from build123d import *

# Parameters (mm, degrees)
F0_R     = 5.5
F1_DEPTH = 9
F3_DEPTH = 9
F4_R     = 7
F5_DEPTH = 9


with BuildPart() as f1:
    # F0 (on Top) → F1 (new body)
    with BuildSketch(Plane.XY):
        with BuildLine():
            Line((-46, 15), (-46, 0))
            ThreePointArc((-46, 0), (-42.192388, -9.192388), (-33, -13))
            Line((-33, -13), (0, -13))
            ThreePointArc((0, -13), (9.192388, -9.192388), (13, 0))
            Line((13, 0), (13, 15))
            Line((13, 15), (-46, 15))
        make_face()
        with Locations((-33, 0)):
            Circle(F0_R, mode=Mode.SUBTRACT)
        Circle(F0_R, mode=Mode.SUBTRACT)
    extrude(amount=F1_DEPTH)

    # F2 (on face) → F3 (join)
    with BuildSketch(Plane(origin=(0, 15, 0), x_dir=(-1, 0, 0), z_dir=(0, 1, 0))):
        Polygon((46, 0), (46, 9), (-20.313708, 75.313708), (-42.941125, 52.686292), (-13, 0), align=None)
    extrude(amount=F3_DEPTH)

    # F4 (on face) → F5 (join)
    with BuildSketch(Plane(origin=(47.813708, 0, 47.813708), x_dir=(0.707107, 0, -0.707107), z_dir=(0.707107, 0, 0.707107))):
        with BuildLine():
            Line((-6.890873, 15), (-6.890873, 24))
            Line((-6.890873, 24), (-38.890873, 24))
            Line((-38.890873, 24), (-38.890873, 15))
            Line((-38.890873, 15), (-38.890875, -5))
            ThreePointArc((-38.890875, -5), (-22.890875, -21), (-6.890875, -5))
            Line((-6.890875, -5), (-6.890873, 15))
        make_face()
        with Locations((-22.890875, -5)):
            Circle(F4_R, mode=Mode.SUBTRACT)
    extrude(amount=F5_DEPTH)


solid = f1.part
For this review, take the finished solid that the model builds, in its own axes (mm). A direction names the side the tool comes from. Round coordinates to 2 decimals unless told otherwise and drop trailing zeros. Order: outer loops, then holes, each group sorted by start corner. A loop starts at its lowest first (then second) coordinate and runs counter-clockwise, first axis right, second up. Notation, with made-up numbers: (37, 49.5) -> (72, 49.5) arc R21 cw to (72, 71.5) -> close; hole circle Ø6 at (30, -4.75). An arc over 180 degrees is marked (long way). Put each result on its own line as item: value.
Q1. Machinability: for faces 4 (the flat face through (-17, 1, 9)), 5 (the flat face through (-16, 5, 0)), 6 (the flat face through (28.955, 1.252, 66.673)), 7 (the flat face through (13, 7, 4)), 8 (the cylindrical face through (30.84, -9.26, 71.07)), which of the approach directions +Z, -Z, +X, -X, +Y, -Y give a long, thin tool a straight path to every point of the face, cutting with its end or side? Answer none if there is none.
Check result:
face 4: +Z, +X, -X, -Y
face 5: -Z, +X, -X, +Y, -Y
face 6: -Z, -X, -Y
face 7: +Z, -Z, +X, -Y
face 8: none
Q2. For probe 1 along Y at (x, z) = (-33, 7); probe 2 along Z at (x, y) = (-16, -1); probe 3 along Z at (x, y) = (43, -12.5), list the stretches that pass through material, from the lowest coordinate up. Write a range as [from, to].
Check result:
probe 1: [-13, -5.5], [5.5, 24]
probe 2: [0, 9]
probe 3: [55.39, 65.36]
Q3. Add section D-D on z = 33.5. Write out the cut boundary in (x, y).
Check result:
outline: (-21.5, 15) -> (32.04, 15) -> (32.04, 24) -> (-21.5, 24) -> close
Q4. Add section A-A on y = 10. Write out the cut boundary in (x, z), plus the area to 3 significant figures.
Check result:
outline: (-46, 0) -> (13, 0) -> (13, 9) -> (-46, 9) -> close; (20.31, 75.31) -> (42.94, 52.69) -> (49.31, 59.05) -> (26.68, 81.68) -> close
area: 819 mm2
Q5. Add section C-C on x = -25. Write out the cut boundary in (y, z).
Check result:
outline: (-13, 0) -> (24, 0) -> (24, 30) -> (15, 30) -> (15, 9) -> (-13, 9) -> close
Q6. Add section B-B on z = 6. Write out the cut boundary in (x, y), plus the area to 3 significant figures.
Check result:
outline: (-46, 0) arc R13 ccw to (-33, -13) -> (0, -13) arc R13 ccw to (13, 0) -> (13, 15) -> (16.41, 15) -> (16.41, 24) -> (-46, 24) -> close; hole circle Ø11 at (-33, 0); hole circle Ø11 at (0, 0)
area: 1,950 mm2
Q7. Insertion check: pin 1 Ø8 at (y, z) = (8, 15.5) entering from -X; pin 2 Ø10 at (y, z) = (6, 52.5) entering from -X; pin 3 Ø2.5 at (x, z) = (-15.5, 2.5) entering from -Y; pin 4 Ø12 at (y, z) = (-9, 50.5) entering from -X. Each pin has a flat end and moves straight along its axis. Give the tip position at first contact, or say it passes through.
Check result:
pin 1: through
pin 2: x = 38.13
pin 3: y = -13
pin 4: x = 39.13
Q8. Mouldability with a two-part tool opening along Y and no side actions: class faces 1 (the flat face through (-17, -13, 4)), 2 (the cylindrical face through (-1.19, -5.37, 4.44)), 3 (the flat face through (37.833, 6.815, 70.522)) as pulls with the +Y half, pulls with the -Y half, needs draft (parallel to the pull), parting line crosses it, or undercut.
Check result:
face 1: pulls with the -Y half
face 2: undercut
face 3: needs draft
